Source: CAD feature listing. Evaluate the final solid. Frame: model axes, mm. Face numbers are marked on the shaded views. A direction names the side the tool comes from. Round coordinates to 2 decimals unless told otherwise and drop trailing zeros. Order: outer loops, then holes, each group sorted by start corner. A loop starts at its lowest first (then second) coordinate and runs counter-clockwise, first axis right, second up. Notation, with made-up numbers: (21.5, -27) -> (35.5, -27) arc R32 ccw to (35.5, -1) -> close; hole circle Ø5 at (6.25, -13). An arc over 180 degrees is marked (long way). Write item = value, one per line. Start each with the question number.
(1) Contact query for flat-ended pins moving along their axis: pin 1 Ø12 at (y, z) = (-7.5, -9.5) entering from +X; pin 2 Ø12 at (x, z) = (-8.5, 0) entering from -Y; pin 3 Ø5 at (y, z) = (0, -13.5) entering from +X. Output: stop coordinate, or through.
(2) Cut plane A-A on z = -1.75. Return the cut outline in (x, y).
(3) Cut plane B-B on z = -10. Return the cut outline in (x, y).
(4) Reachability of the marked faces 4, 5 and 6 from +Z, -Z, +X, -X, +Y, -Y: full face, straight path, thin tool, end or side. Return the list, or none.
(5) Ray query, line 1 (Y direction, x = 0, z = -2.5); line 2 (Z direction, x = -4.5, y = 4); line 3 (Z direction, x = -6.5, y = 4.5). Return the intervals inside material, ascending.
(6) Draft query along Y for the marked faces 1, 2 and 3. Return one class per face: released by +Y, released by -Y, zero draft, split by the parting line, or undercut.
from build123d import *

# Parameters (mm, degrees)
F1_DEPTH  = 4
F2_COUNT  = 9
F4_R      = 1.5
F5_DEPTH  = 4
F6_R      = 5
F7_DEPTH  = 20
F8_DEPTH  = 4
F10_DEPTH = 6
F11_DEPTH = 2.5
F12_R     = 1
F13_R     = 7.5
F13_R_2   = 5
F14_DEPTH = 1


with BuildPart() as f1:
    # F0 (on Top) → F1 (new body)
    with BuildSketch(Plane.XY):
        with BuildLine():
            Line((8.3050784754, 3.467805), (0, 0))
            Line((0, 0), (8.3050784754, -3.467805))
            ThreePointArc((8.3050784754, -3.467805), (8.4643613218, -3.0585270007), (8.6034885901, -2.6419659499))
            ThreePointArc((8.6034885901, -2.6419659499), (9.047405848, -2.0765477235), (9.7559177746, -1.9550110935))
            Line((9.7559177746, -1.9550110935), (9.805066286, -1.9648600782))
            ThreePointArc((9.805066286, -1.9648600782), (11.1634165035, -2.0017278276), (12.4557678163, -1.5818437618))
            ThreePointArc((12.4557678163, -1.5818437618), (12.8193292248, -1.2554624828), (12.9848699654, -0.7957909694))
            Line((12.9848699654, -0.7957909694), (13.0638203653, 0))
            Line((13.0638203653, 0), (12.9848699654, 0.7957909694))
            ThreePointArc((12.9848699654, 0.7957909694), (12.8193292248, 1.2554624828), (12.4557678163, 1.5818437618))
            ThreePointArc((12.4557678163, 1.5818437618), (11.1634165035, 2.0017278276), (9.805066286, 1.9648600782))
            Line((9.805066286, 1.9648600782), (9.7559177746, 1.9550110935))
            ThreePointArc((9.7559177746, 1.9550110935), (9.047405848, 2.0765477235), (8.6034885901, 2.6419659499))
            ThreePointArc((8.6034885901, 2.6419659499), (8.4643613218, 3.0585270007), (8.3050784754, 3.467805))
        make_face()
    extrude(amount=F1_DEPTH)


with BuildPart() as f2_1:
    # F2: instance of F1
    add(f1.part.rotate(Axis((0, 0, 2), (0, 0, -1)), 1 * 360 / F2_COUNT))


with BuildPart() as f2_2:
    # F2: instance of F1
    add(f1.part.rotate(Axis((0, 0, 2), (0, 0, -1)), 2 * 360 / F2_COUNT))


with BuildPart() as f2_3:
    # F2: instance of F1
    add(f1.part.rotate(Axis((0, 0, 2), (0, 0, -1)), 3 * 360 / F2_COUNT))


with BuildPart() as f2_4:
    # F2: instance of F1
    add(f1.part.rotate(Axis((0, 0, 2), (0, 0, -1)), 4 * 360 / F2_COUNT))


with BuildPart() as f2_5:
    # F2: instance of F1
    add(f1.part.rotate(Axis((0, 0, 2), (0, 0, -1)), 5 * 360 / F2_COUNT))


with BuildPart() as f2_6:
    # F2: instance of F1
    add(f1.part.rotate(Axis((0, 0, 2), (0, 0, -1)), 6 * 360 / F2_COUNT))


with BuildPart() as f2_7:
    # F2: instance of F1
    add(f1.part.rotate(Axis((0, 0, 2), (0, 0, -1)), 7 * 360 / F2_COUNT))


with BuildPart() as f2_8:
    # F2: instance of F1
    add(f1.part.rotate(Axis((0, 0, 2), (0, 0, -1)), 8 * 360 / F2_COUNT))


with BuildPart() as f2_7_1:
    add(f2_7.part)

    # F3: union F2_6, F2_4, F2_5, F1, F2_1, F2_3, F2_2, F2_8
    add(f2_6.part)
    add(f2_4.part)
    add(f2_5.part)
    add(f1.part)
    add(f2_1.part)
    add(f2_3.part)
    add(f2_2.part)
    add(f2_8.part)

    # F4 (on face) → F5 (cut, through all)
    with BuildSketch(Plane.XY.offset(4)):
        Circle(F4_R)
    extrude(amount=-F5_DEPTH, mode=Mode.SUBTRACT)

    # F6 (on face) → F7 (join)
    with BuildSketch(Plane(origin=(0, 0, 0), x_dir=(1, 0, 0), z_dir=(0, 0, -1))):
        Circle(F6_R)
    extrude(amount=F7_DEPTH)

    # F8 (cut): a face of the model
    f8_faces = [f2_7_1.faces().sort_by_distance(p)[0] for p in [
        (0, 0, 0),
    ]]
    extrude(f8_faces, amount=-F8_DEPTH, mode=Mode.SUBTRACT)

    # F9 (on Front) → F10 (cut, up to face)
    with BuildSketch(Plane.XZ):
        Polygon((3, -12), (0, -12), (-3, -12), (-3, -18), (3, -18), align=None)
    extrude(amount=-F10_DEPTH, mode=Mode.SUBTRACT)

    # F11 (cut): a face of the model
    f11_faces = [f2_7_1.faces().sort_by_distance(p)[0] for p in [
        (0, 0, -15),
    ]]
    extrude(f11_faces, amount=-F11_DEPTH, mode=Mode.SUBTRACT)

    # F12
    f12_edges = [f2_7_1.edges().sort_by_distance(p)[0] for p in [
        (-5, 0, -20),
    ]]
    fillet(f12_edges, radius=F12_R)

    # F13 (on face) → F14 (join)
    with BuildSketch(Plane(origin=(0, 0, 0), x_dir=(1, 0, 0), z_dir=(0, 0, -1))):
        Circle(F13_R)
        Circle(F13_R_2, mode=Mode.SUBTRACT)
    extrude(amount=F14_DEPTH)


solid = f2_7_1.part
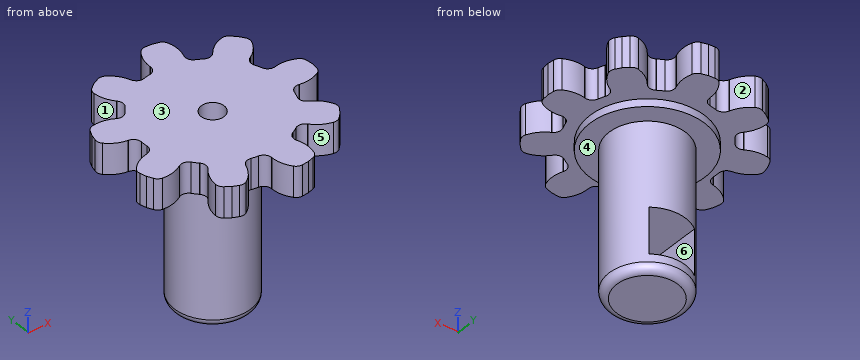
Evaluation:
q1.pin_1 = 4.77
q1.pin_2 = -11.73
q1.pin_3 = 5
q2.outline = circle Ø10 at (0, 0); hole circle Ø3 at (0, 0)
q3.outline = circle Ø10 at (0, 0)
q4.face_4 = -Z
q4.face_5 = +Z, -Z, -Y
q4.face_6 = +Y
q5.line_1 = -5 to -1.5, 1.5 to 5
q5.line_2 = -1 to 4
q5.line_3 = 0 to 4
q6.face_1 = undercut
q6.face_2 = released by +Y
q6.face_3 = zero draft
